Source: CAD feature listing. Evaluate the final solid. Frame: model axes, mm. Face numbers are marked on the shaded views. A direction names the side the tool comes from. Give positions to 0.01 mm unless a question says otherwise; leave off trailing zeros. Order: outer loops, then holes, each group sorted by start corner. A loop starts at its lowest first (then second) coordinate and runs counter-clockwise, first axis right, second up. Notation, with made-up numbers: M 70.5,-18.75 L 76.5,-18.75 A20 ccw 76.5,-2.75 Z; hole C -28.75,-25.75 d8. An arc over 180 degrees is marked long. Return JSON: item names as keys, results as strings.
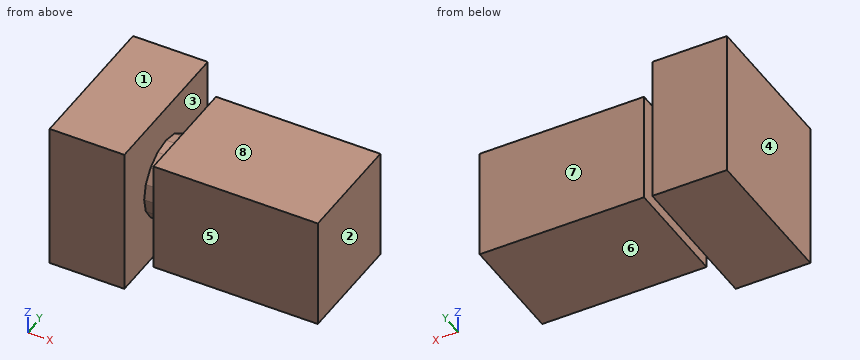
from build123d import *

# Parameters (mm, degrees)
SK_HEAD_W           = 20
SK_HEAD_H           = 40
HEAD_DEPTH          = 40
BUSHING_DEPTH       = 6
SK_CONTACT_BLOCK_W  = 44
SK_CONTACT_BLOCK_H  = 30
CONTACT_BLOCK_DEPTH = 30


with BuildPart() as part:
    # SK_Head → Head (new body)
    with BuildSketch(Plane.XY.offset(215)):
        with Locations((-84, 0)):
            Rectangle(SK_HEAD_W, SK_HEAD_H)
    extrude(amount=HEAD_DEPTH)

    # SK_Bushing → Bushing (add)
    with BuildSketch(Plane(origin=(-74.5, 0, 0), x_dir=(0, 0, -1), z_dir=(1, 0, 0))):
        Polygon((-239.01817604, 9.700735091), (-242.424621202, 7.424621202), (-244.700735091, 4.01817604), (-245.5, 0), (-244.700735091, -4.01817604), (-242.424621202, -7.424621202), (-239.01817604, -9.700735091), (-235, -10.5), (-230.98182396, -9.700735091), (-227.575378798, -7.424621202), (-225.299264909, -4.01817604), (-224.5, 0), (-225.299264909, 4.01817604), (-227.575378798, 7.424621202), (-230.98182396, 9.700735091), (-235, 10.5), align=None)
    extrude(amount=BUSHING_DEPTH)

    # SK_Contact_Block → Contact_Block (add)
    with BuildSketch(Plane.XY.offset(220)):
        with Locations((-47, 0)):
            Rectangle(SK_CONTACT_BLOCK_W, SK_CONTACT_BLOCK_H)
    extrude(amount=CONTACT_BLOCK_DEPTH)


solid = part.part
1. Section query B-B (z = 223). Return loops of the section in (x, y).
Evaluation:
{"outline": "M -94,-20 L -74,-20 L -74,20 L -94,20 Z; M -69,-15 L -25,-15 L -25,15 L -69,15 Z"}
2. First-contact query: pin 1 (9 mm diameter, centred on x = -40, z = 231, fed in from +Y); pin 2 (15 mm diameter, centred on x = -37, z = 234.5, fed in from -Y); pin 3 (24 mm diameter, centred on x = -47.5, y = 6, fed in from -Z). Flat tips, straight axial feed; report the tip coordinate or a pass-through.
Evaluation:
{"pin 1": "stops at y = 15", "pin 2": "stops at y = -15", "pin 3": "stops at z = 220"}
3. Set-up query: the marked faces 5, 6, 7 and 8. Return all of +Z, -Z, +X, -X, +Y, -Y with unobstructed straight access to the full face (end or side cutting, diameter ignored); none if empty.
Evaluation:
{"face 5": "+Z, -Z, +X, -Y", "face 6": "-Z, +X, +Y, -Y", "face 7": "+Z, -Z, +X, +Y", "face 8": "+Z, +X, +Y, -Y"}
4. Section query C-C (x = -70). Return loops of the section in (y, z).
Evaluation:
{"outline": "M -10.5,235 L -9.7,230.98 L -7.42,227.58 L -4.02,225.3 L 0,224.5 L 4.02,225.3 L 7.42,227.58 L 9.7,230.98 L 10.5,235 L 9.7,239.02 L 7.42,242.42 L 4.02,244.7 L 0,245.5 L -4.02,244.7 L -7.42,242.42 L -9.7,239.02 Z"}
5. Draft query along X for the marked faces 1, 2, 3 and 4. Return one class per face: pulls with the +X half, pulls with the -X half, needs draft (parallel to the pull), parting line crosses it, or undercut.
Evaluation:
{"face 1": "needs draft", "face 2": "pulls with the +X half", "face 3": "undercut", "face 4": "pulls with the -X half"}
6. Ray query, probe 1 along X at (y, z) = (2.5, 245.5); probe 2 along Y at (x, z) = (-55.5, 248); probe 3 along X at (y, z) = (-16, 248). Return the intervals inside material, ascending.
Evaluation:
{"probe 1": "x = -94 to -74, -69 to -25", "probe 2": "y = -15 to 15", "probe 3": "x = -94 to -74"}
7. Section query A-A (y = 13.5). Return loops of the section in (x, z).
Evaluation:
{"outline": "M -94,215 L -74,215 L -74,255 L -94,255 Z; M -69,220 L -25,220 L -25,250 L -69,250 Z"}
8. Section query D-D (z = 251.5). Return loops of the section in (x, y), then the cut area to 3 significant figures.
Evaluation:
{"outline": "M -94,-20 L -74,-20 L -74,20 L -94,20 Z", "area": "800 mm^2"}
